```python
from build123d import *

# Parameters (mm, degrees)
SKETCH1_W           = 100
SKETCH1_H           = 5
BOSS_EXTRUDE1_DEPTH = 10
SKETCH2_R           = 3
CUT_EXTRUDE3_DEPTH  = 4
SKETCH3_R           = 1.5
CUT_EXTRUDE4_DEPTH  = 7


with BuildPart() as part:
    # Sketch1 → Boss-Extrude1 (new body)
    with BuildSketch(Plane.XY):
        Rectangle(SKETCH1_W, SKETCH1_H)
    extrude(amount=BOSS_EXTRUDE1_DEPTH)

    # Sketch2 → Cut-Extrude3 (cut)
    with BuildSketch(Plane(origin=(0, 0, 0), x_dir=(-1, 0, 0), z_dir=(0, 0, -1))):
        with Locations((-42, 0)):
            Circle(SKETCH2_R)
        with Locations((42, 0)):
            Circle(SKETCH2_R)
    extrude(amount=-CUT_EXTRUDE3_DEPTH, mode=Mode.SUBTRACT)

    # Sketch3 → Cut-Extrude4 (cut, through all)
    with BuildSketch(Plane(origin=(0, 0, 4), x_dir=(-1, 0, 0), z_dir=(0, 0, -1))):
        with Locations((-42, 0)):
            Circle(SKETCH3_R)
        with Locations((42, 0)):
            Circle(SKETCH3_R)
    extrude(amount=-CUT_EXTRUDE4_DEPTH, mode=Mode.SUBTRACT)


solid = part.part
```
Input: part model. Units: mm. Frame: model coordinates. A direction names the side the tool comes from. Give positions to 0.01 mm unless a question says otherwise; leave off trailing zeros. Order: outer loops, then holes, each group sorted by start corner. A loop starts at its lowest first (then second) coordinate and runs counter-clockwise, first axis right, second up. Notation, with made-up numbers: (-19, 3.25) - (-2, 3.25) arc R25 ccw to (-2, 32.25) - close; hole circle Ø4 at (27.25, 22). An arc over 180 degrees is marked (long way). Put each result on its own line as item: value.
Item 1: Section query B-B, the plane y = 0. Return loops of the section in (x, z), then the cut area to 3 significant figures.
Found:
outline: (-50, 0) - (-45, 0) - (-45, 4) - (-43.5, 4) - (-43.5, 10) - (-50, 10) - close; (-40.5, 4) - (-39, 4) - (-39, 0) - (39, 0) - (39, 4) - (40.5, 4) - (40.5, 10) - (-40.5, 10) - close; (43.5, 4) - (45, 4) - (45, 0) - (50, 0) - (50, 10) - (43.5, 10) - close
area: 916 mm^2
Item 2: Contact query for a flat-ended pin moving along its axis: pin 1 (1.5 mm diameter, centred on x = 42, y = 1, fed in from -Z). Output: stop coordinate, or through.
Found:
pin 1: stops at z = 4
Item 3: Section query A-A, the plane x = -42. Return loops of the section in (y, z).
Found:
outline: (-2.5, 4) - (-1.5, 4) - (-1.5, 10) - (-2.5, 10) - close; (1.5, 4) - (2.5, 4) - (2.5, 10) - (1.5, 10) - close
Item 4: Section query C-C, the plane z = 3. Return loops of the section in (x, y), then the cut area to 3 significant figures.
Found:
outline: (-50, -2.5) - (-43.66, -2.5) arc R3 cw to (-43.66, 2.5) - (-50, 2.5) - close; (-40.34, -2.5) - (40.34, -2.5) arc R3 cw to (40.34, 2.5) - (-40.34, 2.5) arc R3 cw to start; (43.66, -2.5) - (50, -2.5) - (50, 2.5) - (43.66, 2.5) arc R3 cw to start
area: 448 mm^2
Item 5: Section query D-D, the plane z = 8.75. Return loops of the section in (x, y).
Found:
outline: (-50, -2.5) - (50, -2.5) - (50, 2.5) - (-50, 2.5) - close; hole circle Ø3 at (-42, 0); hole circle Ø3 at (42, 0)
Item 6: Draft query along X for faces 3 (the flat face through (-50, 0, 5)), 4 (the cylindrical face through (39, 0, 2)), 5 (the flat face through (-1, 0, 10)). Return one class per face: +X half, -X half, draft (parallel to the pull), parting line (faces both ways), or undercut.
Found:
face 3: -X half
face 4: undercut
face 5: draft
Item 7: Access query for faces 1 (the cylindrical face through (-40.5, 0.07, 6.96)), 2 (the flat face through (-42, -2, 4)). Directions: +Z, -Z, +X, -X, +Y, -Y. A direction counts if a zero-diameter tool reaches every point of the face in a straight line with its end or side. Return the directions, or none.
Found:
face 1: +Z, -Z
face 2: -Z
Item 8: Ray query, L1, parallel to X at y = -0.2, z = 3.5; L2, parallel to X at y = 0.05, z = 6.5; L3, parallel to Y at x = 42, z = 6.9. Return the intervals inside material, ascending. Write a range as from..to.
Found:
L1: x = -50..-44.99, -39.01..39.01, 44.99..50
L2: x = -50..-43.5, -40.5..40.5, 43.5..50
L3: y = -2.5..-1.5, 1.5..2.5
